Autodesk Inventor part; units mm, degrees
ref_plane "YZ Plane" through (0, 0, 0) normal (1, 0, 0) x (0, 1, 0)
ref_plane "XZ Plane" through (0, 0, 0) normal (0, 1, 0) x (-1, 0, 0)
ref_plane "XY Plane" through (0, 0, 0) normal (0, 0, 1) x (1, 0, 0)
sketch "スケッチ1" plane through (0, 0, 0) normal (0, 1, 0) x (-1, 0, 0)
  line L0 (0, 0) -> (-300, 0)
  line L1 (-300, 0) -> (-300, -17.5)
  line L2 (-300, -17.5) -> (0, -17.5)
  line L3 (0, -17.5) -> (0, 0)
  dimension "d0" = 300
  dimension "d1" = 17.5
extrude "押し出し1" add sketch "スケッチ1" along normal blind 2
sketch "スケッチ2" plane through (0, 2, 0) normal (0, 1, 0) x (1, 0, 0)
  line L0 (0, 17.5) -> (0, 0)
  line L1 (0, 8.75) -> (300, 8.75)
  line L2 (300, 0) -> (300, 17.5)
  line L3 (0, 8.75) -> (300, 8.75)
  line L4 (300, 8.75) -> (300, 12.5)
  line L5 (300, 12.5) -> (0, 12.5)
  line L6 (0, 12.5) -> (0, 8.75)
  line L7 (0, 0) -> (0, 17.5)
  line L8 (300, 17.5) -> (300, 0)
  line L9 (300, 5) -> (0, 5)
  line L10 (0, 0) -> (300, 0)
  line L11 (300, 0) -> (300, 17.5)
  line L12 (300, 17.5) -> (0, 17.5)
  line L13 (0, 17.5) -> (0, 0)
  point P0 (0, 12.5)
  point P1 (0, 5)
  dimension "d4" = 3.75
extrude "押し出し2" cut sketch "スケッチ2" against normal blind 1 contours L12 L2 L5 L0 | L9 L2 L10 L0
sketch "スケッチ3" plane through (0, 1, 0) normal (0, 1, 0) x (1, 0, 0)
  line L0 (300, 5) -> (300, 12.5)
  line L1 (300, 8.75) -> (0, 8.75)
  line L2 (0, 12.5) -> (0, 5)
  line L3 (0, 5) -> (300, 5)
  line L4 (0, 0) -> (0, 5)
  point P0 (10, 2.75)
  point P1 (10, 14.75)
  point P2 (56.6667, 2.75)
  point P3 (103.3333, 2.75)
  point P4 (150, 2.75)
  point P5 (196.6667, 2.75)
  point P6 (243.3333, 2.75)
  point P7 (290, 2.75)
  point P8 (56.6667, 14.75)
  point P9 (103.3333, 14.75)
  point P10 (150, 14.75)
  point P11 (196.6667, 14.75)
  point P12 (243.3333, 14.75)
  point P13 (290, 14.75)
  dimension "d42" = 10
  dimension "d43" = 6
  dimension "d46" = 46.6667
hole "穴1" at (10, 1, -2.75) at (10, 1, -14.75) at (290, 1, -2.75) at (290, 1, -14.75) at (243.3333, 1, -2.75) at (243.3333, 1, -14.75) at (196.6667, 1, -14.75) at (196.6667, 1, -2.75) at (150, 1, -2.75) at (150, 1, -14.75) at (103.3333, 1, -14.75) at (103.3333, 1, -2.75) at (56.6667, 1, -14.75) at (56.6667, 1, -2.75) direction (0, -1, 0) diameter 3.1 end through all
sketch "スケッチ4" plane through (0, 2, 0) normal (0, 1, 0) x (1, 0, 0)
  line L0 (300, 0) -> (300, 17.5)
  line L1 (300, 8.75) -> (0, 8.75)
  line L2 (0, 12.5) -> (0, 5)
  point P0 (0, 0)
  point P1 (290, 8.75)
  point P2 (278.8, 8.75)
  point P3 (267.6, 8.75)
  point P4 (256.4, 8.75)
  point P5 (245.2, 8.75)
  point P6 (234, 8.75)
  point P7 (222.8, 8.75)
  point P8 (211.6, 8.75)
  point P9 (200.4, 8.75)
  point P10 (189.2, 8.75)
  point P11 (178, 8.75)
  point P12 (166.8, 8.75)
  point P13 (155.6, 8.75)
  point P14 (144.4, 8.75)
  point P15 (133.2, 8.75)
  point P16 (122, 8.75)
  point P17 (110.8, 8.75)
  point P18 (99.6, 8.75)
  point P19 (88.4, 8.75)
  point P20 (77.2, 8.75)
  point P21 (66, 8.75)
  point P22 (54.8, 8.75)
  point P23 (10, 8.75)
  point P24 (43.6, 8.75)
  point P25 (32.4, 8.75)
  point P26 (21.2, 8.75)
  dimension "d23" = 10
  dimension "d26" = 11.2
  dimension "d39" = 10
hole "穴2" at (290, 2, -8.75) at (278.8, 2, -8.75) at (267.6, 2, -8.75) at (256.4, 2, -8.75) at (245.2, 2, -8.75) at (234, 2, -8.75) at (222.8, 2, -8.75) at (211.6, 2, -8.75) at (200.4, 2, -8.75) at (189.2, 2, -8.75) at (178, 2, -8.75) at (166.8, 2, -8.75) at (155.6, 2, -8.75) at (144.4, 2, -8.75) at (133.2, 2, -8.75) at (122, 2, -8.75) at (110.8, 2, -8.75) at (99.6, 2, -8.75) at (88.4, 2, -8.75) at (77.2, 2, -8.75) at (66, 2, -8.75) at (54.8, 2, -8.75) at (10, 2, -8.75) at (43.6, 2, -8.75) at (32.4, 2, -8.75) at (21.2, 2, -8.75) direction (0, -1, 0) diameter 7 depth 8 tip angle 118
equation "\"d0\" = polygon2_len1"
equation "\"d4\" = 0.5 * polygon2_wid2"
properties part number "link2plate2" material "アルミニウム 6061"
CAD build for the part. Positions are in the model's coordinates, mm. A direction names the side the tool comes from. Round coordinates to 2 decimals unless told otherwise and drop trailing zeros. Loops run counter-clockwise (first coordinate to the right, second up) from the corner with the lowest first, then second, coordinate; pieces in that order, holes last. Notation, with made-up numbers: (9.5, -10) - (17.5, -10) arc R18 ccw to (17.5, 21) - close; hole circle Ø6 at (57, 15). An arc over 180 degrees is marked (long way). Return JSON: item names as keys, results as strings. Group by question number.
Q1. Band-saw the part on B-B on x = 189.2. Give the cut face in (y, z).
Q2. Tool access for faces 3 (the face through (148, 1, -3)), 4 (the face through (63.6, 1, -11.3)), 5 (the face through (148, 1, -15)): list every direction of +Z, -Z, +X, -X, +Y, -Y with a clear straight run to the whole face (end or side of a thin tool).
Q3. Two-plate mould, pull along X, no slides. Class faces 1 (the face through (226.217, 0.986, -9.509)), 2 (the face through (185, 2, -9)): +X half, -X half, draft (parallel to the pull), parting line (faces both ways), or undercut.
Q4. Flat gauge pins, fed straight in: pin 1 Ø9 at (x, z) = (189.2, -8.75) entering from +Y; pin 2 Ø4 at (x, z) = (56.67, -2.75) entering from +Y. Where does each tip first touch, or does it go through?
Q5. Band-saw the part on A-A on y = 1.4. Give the number of separate pieces and of enclosed holes in the cut face, plus the area to 3 significant figures.
Q6. Drill centre lines: line 1 along Z through (x, y) = (144.4, 1.55); line 2 along Z through (x, y) = (256.4, 0.4); line 3 along Y through (x, z) = (14, -13). Where is each one in solid material? Low to high. Write a range as [from, to].
Solutions:
{
 "1": {"outline": "(0, -17.5) - (1, -17.5) - (1, -12.5) - (2, -12.5) - (2, -12.25) - (0, -12.25) - close; (0, -5.25) - (2, -5.25) - (2, -5) - (1, -5) - (1, 0) - (0, 0) - close"},
 "2": {"face 3": "+Z, +X, -X, +Y", "face 4": "+Y, -Y", "face 5": "-Z, +X, -X, +Y"},
 "3": {"face 1": "undercut", "face 2": "draft"},
 "4": {"pin 1": "stops at y = 2", "pin 2": "stops at y = 1"},
 "5": {"separate pieces": "1", "enclosed holes": "26", "area": "1,250 mm^2"},
 "6": {"line 1": "z = [-12.5, -12.25], [-5.25, -5]", "line 2": "z = [-17.5, -12.25], [-5.25, 0]", "line 3": "y = [0, 1]"}
}
